The model under review builds one solid part; all positions refer to its coordinate system, in mm. A direction names the side the tool comes from. Round coordinates to 2 decimals unless told otherwise and drop trailing zeros. Order: outer loops, then holes, each group sorted by start corner. A loop starts at its lowest first (then second) coordinate and runs counter-clockwise, first axis right, second up. Notation, with made-up numbers: (14.25, 88) -> (68.25, 88) arc R32 cw to (68.25, 119) -> close; hole circle Ø1 at (48.25, -40). An arc over 180 degrees is marked (long way). Use a Markdown table: item, result. Add a question column.
```python
from build123d import *

# Parameters (mm, degrees)
TAGLIO_ESTRUSIONE1_START      = -2
SCHIZZO2_R                    = 4.5
TAGLIO_ESTRUSIONE1_DEPTH      = 2
FORO_FILETTATO_M3X0_5_1_D     = 2.5
FORO_FILETTATO_M3X0_5_1_DEPTH = 9
FORO_FILETTATO_M3X0_5_1_TIP   = 0.751075774
SCHIZZO5_R                    = 1
TAGLIO_ESTRUSIONE2_DEPTH      = 34.021984674


with BuildPart() as part:
    # Schizzo1 → Rivoluzione1 (revolve)
    with BuildSketch(Plane.XY, mode=Mode.PRIVATE) as rivoluzione1_sk:
        with BuildLine():
            Line((0, 0), (4.5, 0))
            Line((4.5, 0), (4.5, 6.215934246))
            ThreePointArc((4.5, 6.215934246), (4.461941718, 6.489188945), (4.350663738, 6.741644436))
            Line((4.350663738, 6.741644436), (3.104336262, 8.758355564))
            ThreePointArc((3.104336262, 8.758355564), (2.993058282, 9.010811055), (2.955, 9.284065754))
            Line((2.955, 9.284065754), (2.955, 31.7))
            Line((2.955, 31.7), (0, 31.7))
            Line((0, 31.7), (0, 0))
        make_face()
    revolve(rivoluzione1_sk.sketch.rotate(Axis((0, 31.7, 0), (0, -1, 0)), 180), axis=Axis((0, 31.7, 0), (0, -1, 0)))

    # Schizzo2 → Taglio-Estrusione1 (cut)
    with BuildSketch(Plane.XZ.offset(TAGLIO_ESTRUSIONE1_START)):
        with Locations(Location((0, 0, 0), (0, 0, 180))):
            Circle(SCHIZZO2_R)
        Polygon((0, 3.95), (-3.420800345, 1.975), (-3.420800345, -1.975), (0, -3.95), (3.420800345, -1.975), (3.420800345, 1.975), align=None, mode=Mode.SUBTRACT)
    extrude(amount=TAGLIO_ESTRUSIONE1_DEPTH, mode=Mode.SUBTRACT)

    # Foro filettato M3x0.5-1
    with Locations(Plane(origin=(0, 0, 0), x_dir=(-1, 0, 0), z_dir=(0, -1, 0))):
        with Locations((0, 0)):
            Hole(FORO_FILETTATO_M3X0_5_1_D / 2, depth=FORO_FILETTATO_M3X0_5_1_DEPTH)
            with Locations((0, 0, -(FORO_FILETTATO_M3X0_5_1_DEPTH + FORO_FILETTATO_M3X0_5_1_TIP / 2))):  # 118° drill point
                Cone(0, FORO_FILETTATO_M3X0_5_1_D / 2, FORO_FILETTATO_M3X0_5_1_TIP, mode=Mode.SUBTRACT)

    # Schizzo5 → Taglio-Estrusione2 (cut, through all)
    with BuildSketch(Plane(origin=(-1.4775, 0, -2.559105068), x_dir=(-0.8660254037844385, 0, 0.5000000000000004), z_dir=(-0.5000000000000003, 0, -0.8660254037844384))):
        with Locations((0, 16.7)):
            Circle(SCHIZZO5_R)
        with Locations((0, 20.7)):
            Circle(SCHIZZO5_R)
        with Locations((0, 24.7)):
            Circle(SCHIZZO5_R)
        with Locations((0, 28.7)):
            Circle(SCHIZZO5_R)
    extrude(amount=-TAGLIO_ESTRUSIONE2_DEPTH, mode=Mode.SUBTRACT)

    # TaglioSuperficie1
    split(bisect_by=Plane(origin=(0, 27.7, 0), x_dir=(1, 0, 0), z_dir=(0, 1, 0)), keep=Keep.BOTTOM)


solid = part.part
```
Q1. Add section A-A (z = -0.75). State how many separate pieces and enclosed holes the cut face has, then the cut area to 3 significant figures.
Q2. Machinability: for faces 5 (the flat face through (-1.73, 1.01, -2.95)), 6 (the flat face through (3.421, 1, 0)), 7 (the flat face through (1.73, 1.01, 2.95)), 8 (the flat face through (2, 2, -3)), 9 (the flat face through (-1.686, 1.014, 2.976)), which of the approach directions +Z, -Z, +X, -X, +Y, -Y give a long, thin tool a straight path to every point of the face, cutting with its end or side? Answer none if there is none.
Q3. Insertion check: pin 1 (1.5 mm diameter, centred on y = 15.5, z = 2, fed in from -X); pin 2 (5 mm diameter, centred on x = 3.5, z = 2, fed in from +Y); pin 3 (5 mm diameter, centred on y = 4.5, z = 3.5, fed in from +X); pin 4 (0.6 mm diameter, centred on y = 1.5, z = 0, fed in from -X). Each pin has a flat end and moves straight along its axis. Give the tip position at first contact, or say it passes through.
Q4. Mouldability with a two-part tool opening along Y and no side actions: class faces 1 (the cylindrical face through (0.167, 15.724, -0.144)), 2 (the conical face through (0.05, 9.62, 0.21)), 3 (the cylindrical face through (-0.27, 4.56, 1.22)), 4 (the cylindrical face through (-0.42, 23.81, 0.19)) as pulls with the +Y half, pulls with the -Y half, needs draft (parallel to the pull), parting line crosses it, or undercut.
Q5. Add section D-D (y = 8). Write out the cut boundary in (x, z), then the cut area to 3 significant figures.
Q6. Add section B-B (y = 12.5). Write out the cut boundary in (x, z) (3 decimals), then the cut area to 3 significant figures.
Q7. Wall thickness on line 1 (Y direction, x = 1, z = 1.5); line 2 (Z direction, x = 0, y = 6.25); line 3 (Y direction, x = 1.75, z = 1.75): over which ranges is each line inside the solid? List them lowest first. Write a range as [from, to].
Report:
| question | item | result |
|---|---|---|
| 1 | separate pieces | 1 |
| 1 | enclosed holes | 3 |
| 1 | area | 150 mm² |
| 2 | face 5 | -Z, -X, -Y |
| 2 | face 6 | +Z, -Z, +X, -Y |
| 2 | face 7 | +Z, +X, -Y |
| 2 | face 8 | -Y |
| 2 | face 9 | +Z, -X, -Y |
| 3 | pin 1 | stops at x = -2.68 |
| 3 | pin 2 | stops at y = 27.7 |
| 3 | pin 3 | stops at x = 4.39 |
| 3 | pin 4 | stops at x = -3.42 |
| 4 | face 1 | undercut |
| 4 | face 2 | pulls with the -Y half |
| 4 | face 3 | needs draft |
| 4 | face 4 | undercut |
| 5 | outline | circle Ø7.15 at (0, 0); hole circle Ø2.5 at (0, 0) |
| 5 | area | 35.2 mm² |
| 6 | outline | circle Ø5.91 at (0, 0) |
| 6 | area | 27.4 mm² |
| 7 | line 1 | y = [0, 15.71], [17.69, 19.71], [21.69, 23.71], [25.69, 27.7] |
| 7 | line 2 | z = [-4.5, -1.25], [1.25, 4.5] |
| 7 | line 3 | y = [0, 15.93], [17.47, 19.93], [21.47, 23.93], [25.47, 27.7] |
